Source: three-view drawing plus pictorial views. Frame: mm from the lowest corner of the part. A direction names the side the tool comes from. Give positions to 0.01 mm unless a question says otherwise; leave off trailing zeros. Order: outer loops, then holes, each group sorted by start corner. A loop starts at its lowest first (then second) coordinate and runs counter-clockwise, first axis right, second up. Notation, with made-up numbers: (18, 25.5) -> (38, 25.5) arc R19 ccw to (38, 50.5) -> close; hole circle Ø10 at (62.5, 27.25). An arc over 180 degrees is marked (long way). Write item = value, one per line.
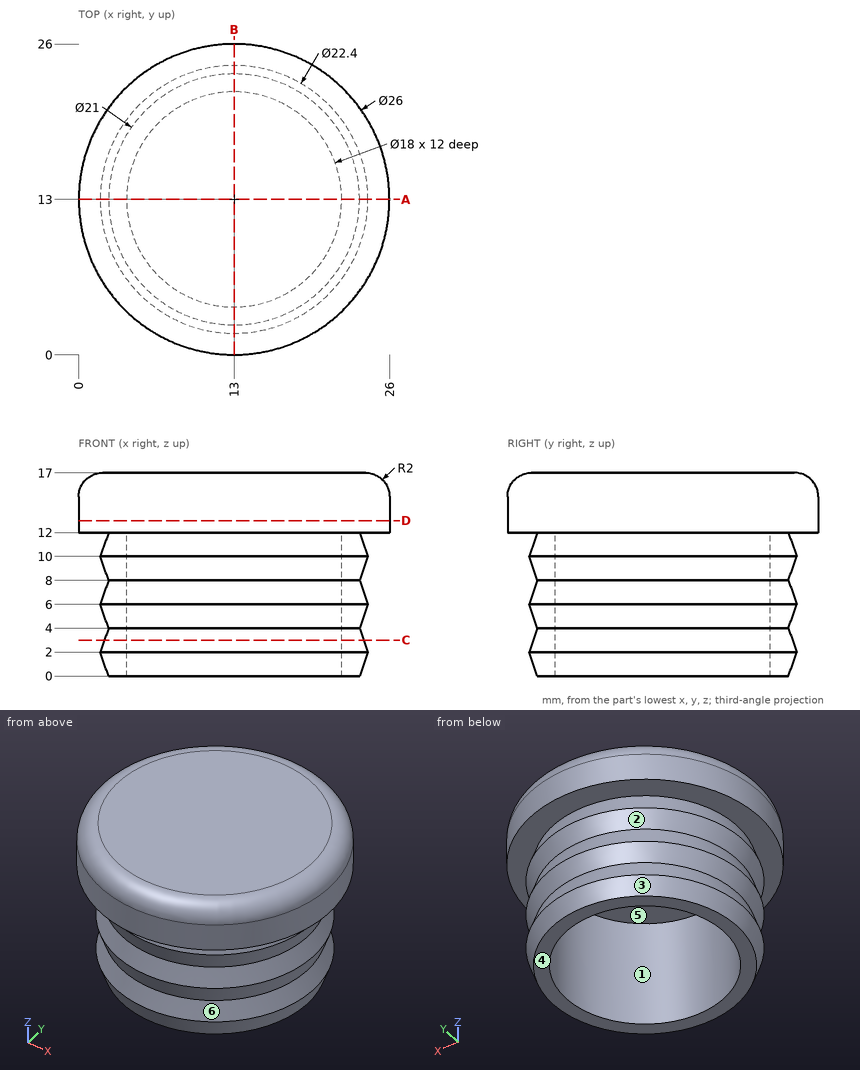
1) Section query D-D (z = 13). Output: boundary loops of the cut face in (x, y).
Check sheet entries:
outline = circle Ø26 at (13, 13)
2) Line query: line 1 (Z direction, x = 18.5, y = 18.5); line 2 (Y direction, x = 13, z = 8.5) (3 decimals); line 3 (Y direction, x = 21.25, z = 5.75). Output: solid intervals per line, ascending. Write a range as from..to.
Check sheet entries:
line_1 = 12..17
line_2 = 2.325..4, 22..23.675
line_3 = 5.56..9.4, 16.6..20.44
3) Reachability of the marked faces 4, 5 and 6 from +Z, -Z, +X, -X, +Y, -Y: full face, straight path, thin tool, end or side. Return the list, or none.
Check sheet entries:
face_4 = -Z, +X, -X, +Y, -Y
face_5 = -Z
face_6 = none
4) Section query A-A (y = 13). Output: boundary loops of the cut face in (x, z).
Check sheet entries:
outline = (0, 12) -> (2.5, 12) -> (1.8, 10) -> (2.5, 8) -> (1.8, 6) -> (2.5, 4) -> (1.8, 2) -> (2.5, 0) -> (4, 0) -> (4, 12) -> (22, 12) -> (22, 0) -> (23.5, 0) -> (24.2, 2) -> (23.5, 4) -> (24.2, 6) -> (23.5, 8) -> (24.2, 10) -> (23.5, 12) -> (26, 12) -> (26, 15) arc R2 ccw to (24, 17) -> (2, 17) arc R2 ccw to (0, 15) -> close
5) Mould query, pull axis Z, two halves, no side actions, for the marked faces 1, 2 and 3. Classes: +Z half, -Z half, draft (parallel to the pull), parting line (faces both ways), or undercut.
Check sheet entries:
face_1 = draft
face_2 = undercut
face_3 = -Z half
6) Section query C-C (z = 3). Output: boundary loops of the cut face in (x, y), plus the area to 3 significant figures.
Check sheet entries:
outline = circle Ø21.7 at (13, 13); hole circle Ø18 at (13, 13)
area = 115 mm²
7) First-contact query: P1, Ø8, axis at x = 17, z = 9, coming from the -Y side; P2, Ø5.5, axis at x = 12.5, y = 9, coming from the -Z side; P3, Ø2, axis at y = 6.5, z = 4, coming from the +X side. Flat tips, straight axial feed; report the tip coordinate or a pass-through.
Check sheet entries:
P1 = 0.07
P2 = 12
P3 = 22.07
